Part model, mm, in its own coordinate system. Give positions to 0.01 mm unless a question says otherwise; leave off trailing zeros. Use a Markdown table: item, result.
Autodesk Inventor part; units mm, degrees
ref_plane "YZ Plane" through (0, 0, 0) normal (1, 0, 0) x (0, 1, 0)
ref_plane "XZ Plane" through (0, 0, 0) normal (0, 1, 0) x (-1, 0, 0)
ref_plane "XY Plane" through (0, 0, 0) normal (0, 0, 1) x (1, 0, 0)
sketch "Esquisse1" plane through (0, 0, 0) normal (0, 0, 1) x (1, 0, 0)
  ellipse E0 centre (-10.6066, 0) end of major axis (-38.5373, 0) minor radius 19.75 (-15.0725, 19.4959) -> (-24.7487, 17.0312) ccw
  ellipse E1 centre (-15.4634, 21.2024) end of major axis (-17.9082, 21.2024) minor radius 1.7287 (-15.0725, 19.4959) -> (-13.2116, 20.529) ccw
  ellipse E2 centre (-10.6066, 19.75) end of major axis (-7.7782, 19.75) minor radius 2 (-8.0016, 20.529) -> (-13.2116, 20.529) ccw
  ellipse E3 centre (-5.7498, 21.2024) end of major axis (-3.305, 21.2024) minor radius 1.7287 (-8.0016, 20.529) -> (-6.1407, 19.4959) ccw
  ellipse E4 centre (-10.6066, 0) end of major axis (17.3241, 0) minor radius 19.75 (3.5355, 17.0312) -> (-6.1407, 19.4959) ccw
  ellipse E5 centre (-10.6066, 0) end of major axis (-38.5373, 0) minor radius 19.75 (-24.7487, -17.0312) -> (-15.0725, -19.4959) ccw
  ellipse E6 centre (-15.4634, -21.2024) end of major axis (-17.9082, -21.2024) minor radius 1.7287 (-13.2116, -20.529) -> (-15.0725, -19.4959) ccw
  ellipse E7 centre (-10.6066, -19.75) end of major axis (-13.435, -19.75) minor radius 2 (-13.2116, -20.529) -> (-8.0016, -20.529) ccw
  ellipse E8 centre (-5.7498, -21.2024) end of major axis (-3.305, -21.2024) minor radius 1.7287 (-6.1407, -19.4959) -> (-8.0016, -20.529) ccw
  ellipse E9 centre (-10.6066, 0) end of major axis (17.3241, 0) minor radius 19.75 (-6.1407, -19.4959) -> (3.5355, -17.0312) ccw
  line L0 (7.3934, 13) -> (-28.6066, 13) construction
  line L1 (-28.6066, 13) -> (-28.6066, -13) construction
  line L2 (-28.6066, -13) -> (7.3934, -13) construction
  line L3 (7.3934, -13) -> (7.3934, 13) construction
  line L4 (7.3934, 13) -> (-28.6066, -13) construction
  line L5 (-28.6066, 13) -> (7.3934, -13) construction
  arc A0 (-31.6066, -11.1719) -> (-24.7487, -17.0312) centre (-9.517, 7.7394) ccw
  line L6 (-31.6066, -11.1719) -> (-31.6066, 0)
  line L7 (-10.6066, 0) -> (-8.2165, 0)
  line L8 (-10.6066, 0) -> (-10.6066, -5.4794)
  arc A1 (-24.7487, 17.0312) -> (-31.6066, 11.1719) centre (-9.517, -7.7394) ccw
  line L9 (-31.6066, 11.1719) -> (-31.6066, 0)
  arc A2 (3.5355, -17.0312) -> (10.3934, -11.1719) centre (-11.6962, 7.7394) ccw
  line L10 (10.3934, -11.1719) -> (10.3934, 0)
  arc A3 (10.3934, 11.1719) -> (3.5355, 17.0312) centre (-11.6962, -7.7394) ccw
  line L11 (10.3934, 11.1719) -> (10.3934, 0)
  point P0 (0, 0)
  point P1 (4.4659, -19.4959)
  point P2 (-4.4659, -19.4959)
  point P3 (14.1421, -17.0312)
  point P4 (14.1421, 17.0312)
  point P5 (-14.1421, -17.0312)
  point P6 (21, 6.606)
  point P7 (14.1424, -17.0311)
  point P8 (14.1419, 17.0313)
  point P9 (0, 19.0996)
  point P10 (-6.6399, 19.0242)
  point P11 (-7.0711, 19.1066)
  point P12 (-14.1418, 17.0314)
  point P13 (21, -6.606)
  dimension "d0" = 36
  dimension "d1" = 26
  dimension "d2" = 29.079
  dimension "d3" = 3
extrude "Extrusion1" add sketch "Esquisse1" along normal blind 2
fillet "Congé1" radius 3 4 edges at (-31.6066, 11.1719, 1) (-31.6066, -11.1719, 1) (10.3934, 11.1719, 1) (10.3934, -11.1719, 1)
sketch "Esquisse4" plane through (0, 0, 0) normal (0, 0, -1) x (-1, 0, 0)
  ellipse E0 centre (10.6066, 19.75) end of major axis (7.7782, 19.75) minor radius 2 (13.2116, 20.529) -> (8.0016, 20.529) ccw
  circle A0 centre (10.6066, 19.75) radius 1.5
  line L0 (0, 0) -> (14.2006, 0)
  circle A1 centre (10.6066, -19.75) radius 1.5
  dimension "d7" = 3
extrude "Extrusion2" cut sketch "Esquisse4" against normal up to surface (2 mm away)
properties part number "support-miroir"
1. Drill centre lines: L1, parallel to Y at x = 4.5, z = 1.7; L2, parallel to X at y = -15, z = 0.2; L3, parallel to Y at x = 0, z = 1.7. Where is each one in solid material? Low to high.
Findings below:
| item | result |
|---|---|
| L1 | -16.41 to 16.41 |
| L2 | -27.64 to 6.43 |
| L3 | -18.27 to 18.27 |
2. Cut at A-A, the plane z = 1.25. State how many separate pieces and enclosed holes the cut face has, then the cut area to 3 significant figures.
Findings below:
| item | result |
|---|---|
| separate pieces | 1 |
| enclosed holes | 2 |
| area | 1,470 mm2 |
3. Drop flat-ended pins along their axis: P1, Ø2.5, axis at x = -10.61, y = 19.75, coming from the +Z side; P2, Ø3, axis at x = -22, y = -14.5, coming from the -Z side. Give the stop position or say it passes through.
Findings below:
| item | result |
|---|---|
| P1 | through |
| P2 | z = 0 |
4. Two-plate mould, pull along Y, no slides. Class faces 1 (the cylindrical face through (-12.037, -19.299, 0.986)), 2 (the cylindrical face through (10.18, -11.14, 1.01)), 3 (the flat face through (-11, 0, 0)): released by +Y, released by -Y, zero draft, split by the parting line, or undercut.
Findings below:
| item | result |
|---|---|
| face 1 | undercut |
| face 2 | released by -Y |
| face 3 | zero draft |
